Source: three-view drawing plus pictorial views. Frame: mm from the lowest corner of the part. A direction names the side the tool comes from. Coordinates: 2 decimals unless noted, no trailing zeros. Order: outer loops, then holes, each group sorted by start corner. A loop starts at its lowest first (then second) coordinate and runs counter-clockwise, first axis right, second up. Notation, with made-up numbers: M 34.5,89.5 L 65.5,89.5 A33 ccw 65.5,117.5 Z; hole C -23,44 d1. An arc over 180 degrees is marked long. One line per question, with ' | ' between items.
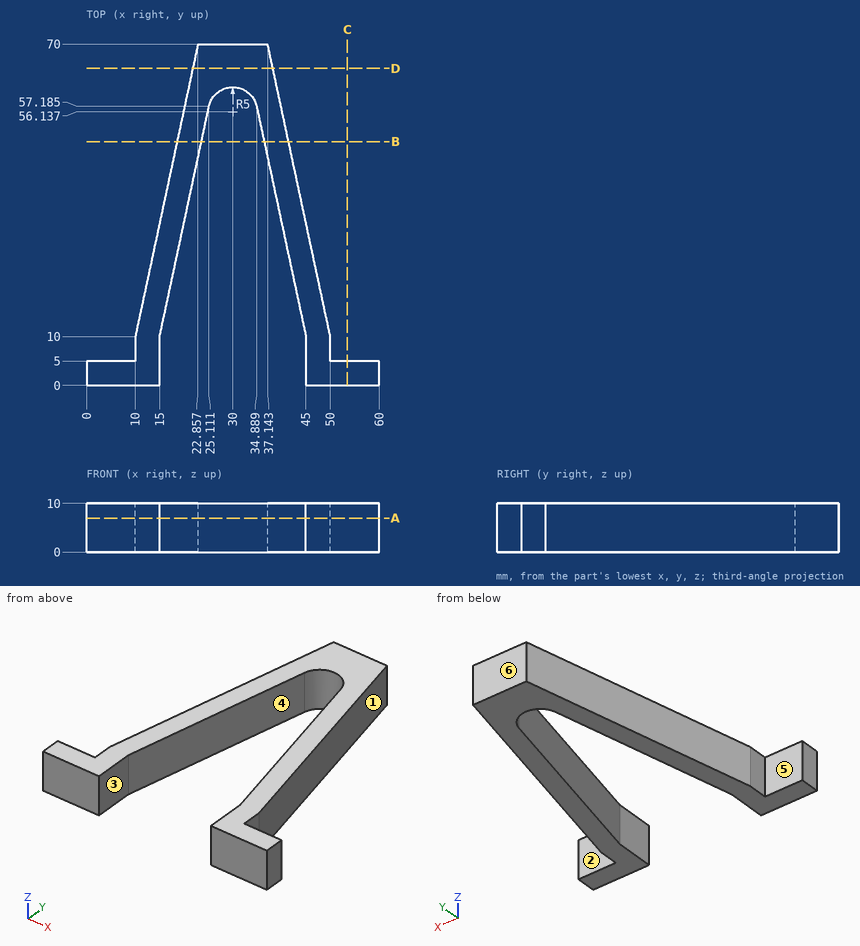
1. Material intervals for line 1 (X direction, y = 6, z = 5.75); line 2 (X direction, y = 37, z = 1.75) (1 decimal); line 3 (Y direction, x = 9.5, z = 8.25), sorted ascending. Write a range as [from, to].
Response values:
line 1: x = [10, 15], [45, 50] | line 2: x = [15.8, 20.8], [39.2, 44.2] | line 3: y = [0, 5]
2. Section B-B, the plane y = 50. Output: boundary loops of the cut face in (x, z), and give its area (4 significant figures).
Response values:
outline: M 18.57,0 L 23.57,0 L 23.57,10 L 18.57,10 Z; M 36.43,0 L 41.43,0 L 41.43,10 L 36.43,10 Z | area: 100.0 mm^2
3. Section A-A, the plane z = 7. Output: boundary loops of the cut face in (x, y) (1 decimal).
Response values:
outline: M 0,0 L 15,0 L 15,10 L 25.1,57.2 A5 cw 34.9,57.2 L 45,10 L 45,0 L 60,0 L 60,5 L 50,5 L 50,10 L 37.1,70 L 22.9,70 L 10,10 L 10,5 L 0,5 Z
4. Draft query along X for the marked faces 1, 2 and 3. Return one class per face: pulls with the +X half, pulls with the -X half, needs draft (parallel to the pull), parting line crosses it, or undercut.
Response values:
face 1: pulls with the +X half | face 2: needs draft | face 3: undercut
5. Section D-D, the plane y = 65. Output: boundary loops of the cut face in (x, z) (1 decimal).
Response values:
outline: M 21.8,0 L 38.2,0 L 38.2,10 L 21.8,10 Z
6. Section C-C, the plane x = 53.5. Output: boundary loops of the cut face in (y, z).
Response values:
outline: M 0,0 L 5,0 L 5,10 L 0,10 Z
7. Access query for the marked faces 4, 5 and 6. Directions: +Z, -Z, +X, -X, +Y, -Y. A direction counts if a zero-diameter tool reaches every point of the face in a straight line with its end or side. Return the directions, or none.
Response values:
face 4: +Z, -Z, -Y | face 5: +Z, -Z, -X, +Y | face 6: +Z, -Z, +X, -X, +Y
8. Pin query (flat end, axial travel): P1, Ø6, axis at x = 46.5, y = 14, coming from the -Z side; P2, Ø1.5, axis at y = 45.5, z = 8.5, coming from the +X side; P3, Ø2, axis at y = 62, z = 7.5, coming from the -X side; P4, Ø4, axis at y = 13, z = 3.5, coming from the +X side. Return the tip coordinate at first contact, or that it passes through.
Response values:
P1: stops at z = 0 | P2: stops at x = 42.55 | P3: stops at x = 20.93 | P4: stops at x = 49.79
